```python
from build123d import *

# Parameters (mm, degrees)
SKETCH1_W                   = 12.7
SKETCH1_H                   = 127
BOSS_EXTRUDE1_DEPTH         = 3.175
F_1_4_0_25_DIAMETER_HOLE1_D = 6.35


with BuildPart() as part:
    # Sketch1 → Boss-Extrude1 (new body)
    with BuildSketch(Plane(origin=(0, 25.4, 0), x_dir=(1, 0, 0), z_dir=(0, 1, 0))):
        with BuildLine():
            Line((-91.44, 342.9), (-101.6, 342.9))
            Line((-101.6, 342.9), (-101.6, 215.9))
            Line((-101.6, 215.9), (98.425, 215.9))
            Line((98.425, 215.9), (101.6, 215.9))
            Line((101.6, 215.9), (101.6, 342.9))
            Line((101.6, 342.9), (91.44, 342.9))
            Line((91.44, 342.9), (91.44, 308.61))
            Line((91.44, 308.61), (91.44, 237.49))
            ThreePointArc((91.44, 237.49), (89.952102448, 233.897897552), (86.36, 232.41))
            Line((86.36, 232.41), (-86.36, 232.41))
            ThreePointArc((-86.36, 232.41), (-89.952102448, 233.897897552), (-91.44, 237.49))
            Line((-91.44, 237.49), (-91.44, 308.61))
            Line((-91.44, 308.61), (-91.44, 342.9))
        make_face()
        with Locations((-107.95, 279.4)):
            Rectangle(SKETCH1_W, SKETCH1_H)
        with Locations((107.95, 279.4)):
            Rectangle(SKETCH1_W, SKETCH1_H)
    extrude(amount=BOSS_EXTRUDE1_DEPTH)

    # 1/4 (0.25) Diameter Hole1 (through all)
    with Locations(Plane(origin=(0, 28.575, 0), x_dir=(1, 0, 0), z_dir=(0, 1, 0))):
        with Locations((101.6, 330.2), (101.6, 222.25), (38.1, 222.25), (-98.802463558, 332.626703007), (-101.416445229, 224.708356097), (-37.935064693, 223.17071982)):
            Hole(F_1_4_0_25_DIAMETER_HOLE1_D / 2)


solid = part.part
```
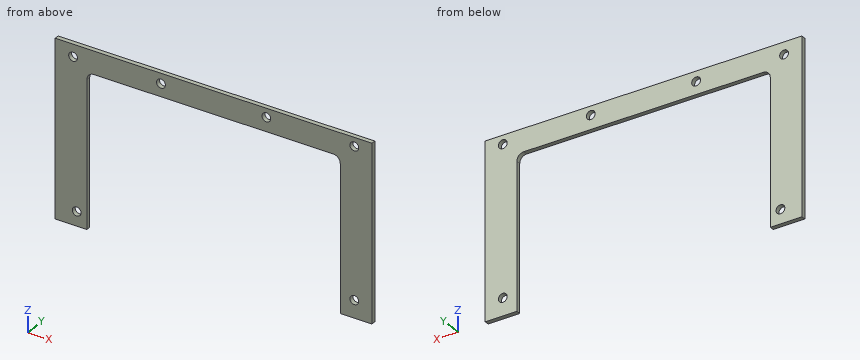
The listing builds one solid part. Answer for the finished solid, in the listing's coordinates (mm). Coordinates: 2 decimals unless noted, no trailing zeros. Loops run counter-clockwise (first coordinate to the right, second up) from the corner with the lowest first, then second, coordinate; pieces in that order, holes last. Notation, with made-up numbers: (32, -4.5) -> (85, -4.5) arc R24 cw to (85, 27.5) -> close; hole circle Ø5 at (-7, 17). An arc over 180 degrees is marked (long way). Return JSON: item names as keys, results as strings. Group by question number.
(1) A cutting plane is placed at B-B on z = -277. Write down the section's boundary in (x, y) (3 decimals), and give its area (3 significant figures).
(2) Find the intervals of material crossed by probe 1 along Z at (x, y) = (101.6, 27.4) (3 decimals); probe 2 along X at (y, z) = (26.3, -284.5); probe 3 along X at (y, z) = (27.75, -222.25) (1 decimal), in increasing order. Write a range as from..to.
(3) A cutting plane is placed at D-D on y = 27.1. Write down the section's boundary in (x, z) (3 decimals).
(4) A cutting plane is placed at A-A on x = 38.1. Write down the section's boundary in (y, z) (3 decimals).
(5) Given pin 1 Ø1 at (x, y) = (-38.5, 26.5) entering from -Z, flat-ended and moving along its own axis, determine where the tip first touches the part or whether it passes through.
(6) A cutting plane is placed at C-C on x = 101.6. Write down the section's boundary in (y, z) (3 decimals).
The answers:
{
 "1": {"outline": "(-114.3, 25.4) -> (-91.44, 25.4) -> (-91.44, 28.575) -> (-114.3, 28.575) -> close; (91.44, 25.4) -> (114.3, 25.4) -> (114.3, 28.575) -> (91.44, 28.575) -> close", "area": "145 mm^2"},
 "2": {"probe 1": "z = -342.9..-333.375, -327.025..-225.425, -219.075..-215.9", "probe 2": "x = -114.3..-91.44, 91.44..114.3", "probe 3": "x = -114.3..-103.4, -99.4..-41, -34.9..34.9, 41.3..98.4, 104.8..114.3"},
 "3": {"outline": "(-114.3, -342.9) -> (-91.44, -342.9) -> (-91.44, -237.49) arc R5.08 cw to (-86.36, -232.41) -> (86.36, -232.41) arc R5.08 cw to (91.44, -237.49) -> (91.44, -342.9) -> (114.3, -342.9) -> (114.3, -215.9) -> (-114.3, -215.9) -> close; hole circle Ø6.35 at (-101.416, -224.708); hole circle Ø6.35 at (-98.802, -332.627); hole circle Ø6.35 at (-37.935, -223.171); hole circle Ø6.35 at (38.1, -222.25); hole circle Ø6.35 at (101.6, -330.2); hole circle Ø6.35 at (101.6, -222.25)"},
 "4": {"outline": "(25.4, -232.41) -> (28.575, -232.41) -> (28.575, -225.425) -> (25.4, -225.425) -> close; (25.4, -219.075) -> (28.575, -219.075) -> (28.575, -215.9) -> (25.4, -215.9) -> close"},
 "5": {"pin 1": "stops at z = -232.41"},
 "6": {"outline": "(25.4, -342.9) -> (28.575, -342.9) -> (28.575, -333.375) -> (25.4, -333.375) -> close; (25.4, -327.025) -> (28.575, -327.025) -> (28.575, -225.425) -> (25.4, -225.425) -> close; (25.4, -219.075) -> (28.575, -219.075) -> (28.575, -215.9) -> (25.4, -215.9) -> close"}
}
